from build123d import *

# Parameters (mm, degrees)
ESQUISSE1_W             = 63
ESQUISSE1_H             = 57
BOSS_EXTRU_1_DEPTH      = 3
ESQUISSE2_W             = 3
ESQUISSE2_H             = 8.333333333
ESQUISSE2_H_2           = 8.333333334
ENL_V_MAT_EXTRU_1_DEPTH = 3
CONG_1_R                = 10


with BuildPart() as part:
    # Esquisse1 → Boss.-Extru.1 (new body)
    with BuildSketch(Plane(origin=(0, 0, 0), x_dir=(1, 0, 0), z_dir=(0, 1, 0))):
        with Locations((-31.5, 28.5)):
            Rectangle(ESQUISSE1_W, ESQUISSE1_H)
    extrude(amount=BOSS_EXTRU_1_DEPTH)

    # Esquisse2 → Enlèv. mat.-Extru.1 (cut)
    with BuildSketch(Plane(origin=(0, 3, 0), x_dir=(1, 0, 0), z_dir=(0, 1, 0))):
        with Locations((-1.5, 12.166666667)):
            Rectangle(ESQUISSE2_W, ESQUISSE2_H)
        with Locations((-1.5, 28.5)):
            Rectangle(ESQUISSE2_W, ESQUISSE2_H_2)
        with Locations((-1.5, 44.833333334)):
            Rectangle(ESQUISSE2_W, ESQUISSE2_H)
    extrude(amount=-ENL_V_MAT_EXTRU_1_DEPTH, mode=Mode.SUBTRACT)

    # Congé1
    cong_1_edges = [part.edges().sort_by_distance(p)[0] for p in [
        (-63, 1.5, 0),
        (-63, 1.5, -57),
    ]]
    fillet(cong_1_edges, radius=CONG_1_R)


solid = part.part
Model file for the job. Use its own axes, mm. A direction names the side the tool comes from. Coordinates: 2 decimals unless noted, no trailing zeros. Loops run counter-clockwise (first coordinate to the right, second up) from the corner with the lowest first, then second, coordinate; pieces in that order, holes last. Notation, with made-up numbers: (47.25, 81.5) -> (99.25, 81.5) arc R29 ccw to (99.25, 113.5) -> close; hole circle Ø2 at (71.5, -2). An arc over 180 degrees is marked (long way). Use one line per item in the form item = value. Start each with the question number.
(1) Tool access for faces 4 (the flat face through (0, 1, -4)), 5 (the flat face through (-2, 2, -24.333)): list every direction of +Z, -Z, +X, -X, +Y, -Y with a clear straight run to the whole face (end or side of a thin tool).
(2) Flat gauge pin, fed straight in: pin 1 (0.9 mm diameter, centred on y = 1.5, z = -29, fed in from +X). Where does the tip first touch, or does it go through?
(3) Pull direction Z, two halves, no side cores. Call faces 1 (the flat face through (-27, 1, -57)), 2 (the flat face through (-32, 0, -29)), 3 (the flat face through (-3, 2, -12)): pulls with the +Z half, pulls with the -Z half, needs draft (parallel to the pull), parting line crosses it, or undercut.
(4) Cut at C-C on x = -59. Give the cut face in (y, z).
(5) Cut at B-B on z = -31.5. Give the cut face in (x, y).
(6) Cut at A-A on y = 1.35. Give the cut face in (x, z).
(7) Probe probe 1 along X at (y, z) = (0.25, -43.5); probe 2 along X at (y, z) = (2.2, -7.5); probe 3 along Z at (x, y) = (-59, 0.9). List the from-to ranges inside material, lowest first. Write a range as from..to.
Values:
q1.face_4 = +Z, -Z, +X, +Y, -Y
q1.face_5 = +X, +Y, -Y
q2.pin_1 = -3
q3.face_1 = pulls with the -Z half
q3.face_2 = needs draft
q3.face_3 = undercut
q4.outline = (0, -55) -> (3, -55) -> (3, -2) -> (0, -2) -> close
q5.outline = (-63, 0) -> (-3, 0) -> (-3, 3) -> (-63, 3) -> close
q6.outline = (-63, -47) arc R10 ccw to (-53, -57) -> (0, -57) -> (0, -49) -> (-3, -49) -> (-3, -40.67) -> (0, -40.67) -> (0, -32.67) -> (-3, -32.67) -> (-3, -24.33) -> (0, -24.33) -> (0, -16.33) -> (-3, -16.33) -> (-3, -8) -> (0, -8) -> (0, 0) -> (-53, 0) arc R10 ccw to (-63, -10) -> close
q7.probe_1 = -63..-3
q7.probe_2 = -62.68..0
q7.probe_3 = -55..-2
